from build123d import *

# Parameters (mm, degrees)
ESQUISSE1_W             = 240
ESQUISSE1_H             = 240
BOSS_EXTRU_1_DEPTH      = 10
ESQUISSE2_R             = 7.25
ENL_V_MAT_EXTRU_1_DEPTH = 10
ESQUISSE5_W             = 20
ESQUISSE5_H             = 40
BOSS_EXTRU_5_DEPTH      = 30
ESQUISSE7_R             = 10.3
ENL_V_MAT_EXTRU_2_DEPTH = 80
CONG_1_R                = 2
CONG_2_R                = 2
CONG_3_R                = 2
CONG_4_R                = 2
CONG_5_R                = 2
CONG_6_R                = 2
CONG_7_R                = 2
CONG_8_R                = 2
CONG_9_R                = 2
CONG_10_R               = 2
CONG_11_R               = 2
CONG_12_R               = 2


with BuildPart() as part:
    # Esquisse1 → Boss.-Extru.1 (new body)
    with BuildSketch(Plane(origin=(0, 0, 0), x_dir=(1, 0, 0), z_dir=(0, 1, 0))):
        Rectangle(ESQUISSE1_W, ESQUISSE1_H)
    extrude(amount=BOSS_EXTRU_1_DEPTH)

    # Esquisse2 → Enlèv. mat.-Extru.1 (cut)
    with BuildSketch(Plane(origin=(0, 10, 0), x_dir=(1, 0, 0), z_dir=(0, 1, 0))):
        with Locations((-95, -95)):
            Circle(ESQUISSE2_R)
        with Locations((-95, 95)):
            Circle(ESQUISSE2_R)
        with Locations((95, 95)):
            Circle(ESQUISSE2_R)
        with Locations((95, -95)):
            Circle(ESQUISSE2_R)
    extrude(amount=-ENL_V_MAT_EXTRU_1_DEPTH, mode=Mode.SUBTRACT)

    # Esquisse5 → Boss.-Extru.5 (add)
    with BuildSketch(Plane(origin=(0, 10, 0), x_dir=(1, 0, 0), z_dir=(0, 1, 0))):
        with Locations((-30, 0)):
            Rectangle(ESQUISSE5_W, ESQUISSE5_H)
        with Locations((30, 0)):
            Rectangle(ESQUISSE5_W, ESQUISSE5_H)
    extrude(amount=BOSS_EXTRU_5_DEPTH)

    # Esquisse7 → Enlèv. mat.-Extru.2 (cut)
    with BuildSketch(Plane.ZY.offset(40)):
        with Locations((0, 25)):
            Circle(ESQUISSE7_R)
    extrude(amount=-ENL_V_MAT_EXTRU_2_DEPTH, mode=Mode.SUBTRACT)

    # Congé1
    cong_1_edges = [part.edges().sort_by_distance(p)[0] for p in [
        (-120, 5, -120),
    ]]
    fillet(cong_1_edges, radius=CONG_1_R)

    # Congé2
    cong_2_edges = [part.edges().sort_by_distance(p)[0] for p in [
        (-120, 5, 120),
    ]]
    fillet(cong_2_edges, radius=CONG_2_R)

    # Congé3
    cong_3_edges = [part.edges().sort_by_distance(p)[0] for p in [
        (120, 5, 120),
    ]]
    fillet(cong_3_edges, radius=CONG_3_R)

    # Congé4
    cong_4_edges = [part.edges().sort_by_distance(p)[0] for p in [
        (120, 5, -120),
    ]]
    fillet(cong_4_edges, radius=CONG_4_R)

    # Congé5
    cong_5_edges = [part.edges().sort_by_distance(p)[0] for p in [
        (30, 40, -20),
    ]]
    fillet(cong_5_edges, radius=CONG_5_R)

    # Congé6
    cong_6_edges = [part.edges().sort_by_distance(p)[0] for p in [
        (30, 40, 20),
    ]]
    fillet(cong_6_edges, radius=CONG_6_R)

    # Congé7
    cong_7_edges = [part.edges().sort_by_distance(p)[0] for p in [
        (40, 24, -20),
        (40, 39.414213562, -19.414213562),
        (40, 40, 0),
        (40, 24, 20),
        (40, 39.414213562, 19.414213562),
    ]]
    fillet(cong_7_edges, radius=CONG_7_R)

    # Congé8
    cong_8_edges = [part.edges().sort_by_distance(p)[0] for p in [
        (-20, 40, 0),
    ]]
    fillet(cong_8_edges, radius=CONG_8_R)

    # Congé9
    cong_9_edges = [part.edges().sort_by_distance(p)[0] for p in [
        (-20, 24, 20),
        (-20.585786438, 39.414213562, 20),
        (-31, 40, 20),
    ]]
    fillet(cong_9_edges, radius=CONG_9_R)

    # Congé10
    cong_10_edges = [part.edges().sort_by_distance(p)[0] for p in [
        (-40, 24, 20),
        (-40, 39.414213562, 19.414213562),
        (-40, 40, -1),
    ]]
    fillet(cong_10_edges, radius=CONG_10_R)

    # Congé11
    cong_11_edges = [part.edges().sort_by_distance(p)[0] for p in [
        (-30, 40, -20),
        (-20, 24, -20),
        (-20.585786438, 39.414213562, -20),
        (-40, 24, -20),
        (-39.414213562, 39.414213562, -20),
    ]]
    fillet(cong_11_edges, radius=CONG_11_R)

    # Congé12
    cong_12_edges = [part.edges().sort_by_distance(p)[0] for p in [
        (20, 40, 0),
        (20, 24, -20),
        (20, 39.414213562, -19.414213562),
        (20, 24, 20),
        (20, 39.414213562, 19.414213562),
    ]]
    fillet(cong_12_edges, radius=CONG_12_R)


solid = part.part
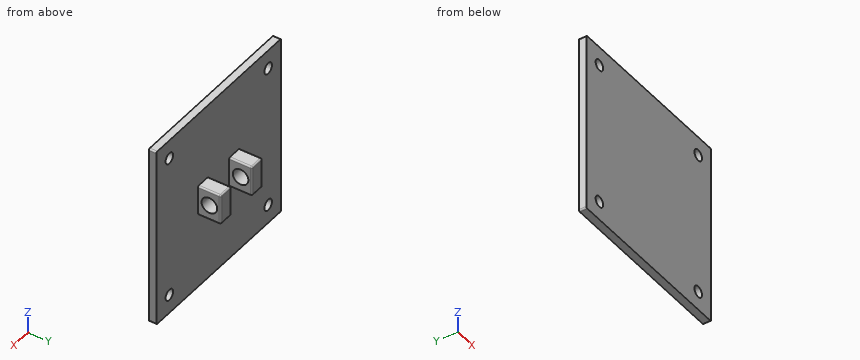
Read the model definition and answer for the solid it produces. Units are mm, in the model's axes. Coordinates: 2 decimals unless noted, no trailing zeros. Order: outer loops, then holes, each group sorted by start corner. A loop starts at its lowest first (then second) coordinate and runs counter-clockwise, first axis right, second up. Notation, with made-up numbers: (28.25, 68) -> (33.25, 68) arc R33 cw to (33.25, 107) -> close; hole circle Ø5 at (39.5, -11.75). An arc over 180 degrees is marked (long way). Answer as a JSON object with one key per item and string values.
1) Consider line 1 along Z through (x, y) = (95, 4); line 2 along X through (y, z) = (38.5, 2). Determine where each line is inside the solid, lowest interval first. Write a range as from..to.
Model answer:
{"line 1": "z = -120..-102.25, -87.75..87.75, 102.25..120", "line 2": "x = -39.94..-20.06, 20.06..39.94"}
2) Each of these flat-tipped pins is pushed along its axis until it touches: pin 1 (8 mm diameter, centred on x = 28, y = 27.5, fed in from -Z); pin 2 (17.5 mm diameter, centred on x = -31.5, y = 22.5, fed in from +Z); pin 3 (6 mm diameter, centred on x = -54, z = 43.5, fed in from +Y). Where does it stop, or does it pass through?
Model answer:
{"pin 1": "stops at z = -20", "pin 2": "stops at z = 20", "pin 3": "stops at y = 10"}
3) A cutting plane is placed at B-B, the plane z = 0. Determine the outline of the cut face in (x, y), plus the area to 3 significant figures.
Model answer:
{"outline": "(-120, 0) -> (120, 0) -> (120, 10) -> (40, 10) -> (40, 14.7) -> (20, 14.7) -> (20, 10) -> (-20, 10) -> (-20, 14.7) -> (-40, 14.7) -> (-40, 10) -> (-120, 10) -> close; (-40, 35.3) -> (-20, 35.3) -> (-20, 38) arc R2 ccw to (-22, 40) -> (-38, 40) arc R2 ccw to (-40, 38) -> close; (20, 35.3) -> (40, 35.3) -> (40, 38) arc R2 ccw to (38, 40) -> (22, 40) arc R2 ccw to (20, 38) -> close", "area": "2,770 mm²"}
4) A cutting plane is placed at A-A, the plane x = 95. Determine the outline of the cut face in (y, z).
Model answer:
{"outline": "(0, -120) -> (10, -120) -> (10, -102.25) -> (0, -102.25) -> close; (0, -87.75) -> (10, -87.75) -> (10, 87.75) -> (0, 87.75) -> close; (0, 102.25) -> (10, 102.25) -> (10, 120) -> (0, 120) -> close"}
5) A cutting plane is placed at D-D, the plane z = 95. Determine the outline of the cut face in (x, y).
Model answer:
{"outline": "(-120, 0) -> (-102.25, 0) -> (-102.25, 10) -> (-120, 10) -> close; (-87.75, 0) -> (87.75, 0) -> (87.75, 10) -> (-87.75, 10) -> close; (102.25, 0) -> (120, 0) -> (120, 10) -> (102.25, 10) -> close"}
6) A cutting plane is placed at C-C, the plane y = 17.5. Determine the outline of the cut face in (x, z).
Model answer:
{"outline": "(-40, -18) arc R2 ccw to (-38, -20) -> (-22, -20) arc R2 ccw to (-20, -18) -> (-20, -7.06) -> (-40, -7.06) -> close; (-40, 7.06) -> (-20, 7.06) -> (-20, 18) arc R2 ccw to (-22, 20) -> (-38, 20) arc R2 ccw to (-40, 18) -> close; (20, -18) arc R2 ccw to (22, -20) -> (38, -20) arc R2 ccw to (40, -18) -> (40, -7.06) -> (20, -7.06) -> close; (20, 7.06) -> (40, 7.06) -> (40, 18) arc R2 ccw to (38, 20) -> (22, 20) arc R2 ccw to (20, 18) -> close"}
